Work out the finished part from the listing and answer in its coordinate system (mm). A direction names the side the tool comes from. Give positions to 0.01 mm unless a question says otherwise; leave off trailing zeros. Order: outer loops, then holes, each group sorted by start corner. A loop starts at its lowest first (then second) coordinate and runs counter-clockwise, first axis right, second up. Notation, with made-up numbers: (63, 26.25) -> (76, 26.25) arc R13 cw to (76, 47.25) -> close; hole circle Ø4 at (83, 57.5). An arc over 180 degrees is marked (long way). Use a Markdown table: item, result. Add a question column.
```python
from build123d import *

# Parameters (mm, degrees)
F1_DEPTH     = 6
F2_W         = 20.4
F2_H         = 50.2
F3_DEPTH     = 4.8
F4_R         = 8
F5_DEPTH     = 10.801
F6_R         = 2.4
F7_DEPTH     = 6.001
F8_R         = 7
F9_R         = 5
F10_T1_DEPTH = 6.0500204163


# Not quite as in the source:
# - a fillet or chamfer that OpenCascade refuses, or shapes differently, is made with other operations: its cross-section is extruded or revolved along the edge and cut away or added


with BuildPart() as f1:
    # F0 (on Top) → F1 (new body)
    with BuildSketch(Plane.XY):
        Polygon((-31, 20), (-31, 0), (31, 0), (31, 20), (17, 20), (17, 50.2), (-17, 50.2), (-17, 20), align=None)
    extrude(amount=F1_DEPTH)

    # F2 (on face) → F3 (join)
    with BuildSketch(Plane.XY.offset(6)):
        with Locations((0, 25.1)):
            Rectangle(F2_W, F2_H)
    extrude(amount=F3_DEPTH)

    # F4 (on face) → F5 (cut, through all)
    with BuildSketch(Plane.XY.offset(10.8)):
        with Locations((0, 33.2)):
            Circle(F4_R)
    extrude(amount=-F5_DEPTH, mode=Mode.SUBTRACT)

    # F6 (on face) → F7 (cut, through all)
    with BuildSketch(Plane.XY.offset(6)):
        with Locations((-25, 10)):
            Circle(F6_R)
        with Locations((25, 10)):
            Circle(F6_R)
    extrude(amount=-F7_DEPTH, mode=Mode.SUBTRACT)

    # F8
    f8_edges = [f1.edges().sort_by_distance(p)[0] for p in [
        (17, 50.2, 3),
        (-17, 50.2, 3),
    ]]
    fillet(f8_edges, radius=F8_R)

    # F9
    f9_edges = [f1.edges().sort_by_distance(p)[0] for p in [
        (-31, 20, 3),
        (31, 20, 3),
        (17, 20, 3),
        (-17, 20, 3),
    ]]
    fillet(f9_edges, radius=F9_R)

    # F10: fillet of radius 0.5 on 2 edges, made by hand

    # F10_s2 → F10_t1 (cut)
    with BuildSketch(Plane.XY.offset(6)):
        with BuildLine():
            ThreePointArc((9.7, 50.2), (10.0535533906, 50.0535533906), (10.2, 49.7))
            Line((10.2, 49.7), (10.25, 49.7))
            Line((10.25, 49.7), (10.25, 50.1971422738))
            Line((10.25, 50.1971422738), (10.2014285714, 50.2471218615))
            ThreePointArc((10.2014285714, 50.2471218615), (10, 50.25), (9.7, 50.25))
            Line((9.7, 50.25), (9.7, 50.2))
        make_face()
        with BuildLine():
            ThreePointArc((-9.7, 50.2), (-10.0535533906, 50.0535533906), (-10.2, 49.7))
            Line((-10.2, 49.7), (-10.25, 49.7))
            Line((-10.25, 49.7), (-10.25, 50.1971422738))
            Line((-10.25, 50.1971422738), (-10.2014285714, 50.2471218615))
            ThreePointArc((-10.2014285714, 50.2471218615), (-10, 50.25), (-9.7, 50.25))
            Line((-9.7, 50.25), (-9.7, 50.2))
        make_face()
    extrude(amount=F10_T1_DEPTH, mode=Mode.SUBTRACT)


solid = f1.part
```
1) Which of the six approach directions +Z, -Z, +X, -X, +Y, -Y give full straight-line access (tool end or side, diameter ignored) to faces 1 (the flat face through (18, 20, 6)), 2 (the flat face through (-18, 20, 6)), 3 (the flat face through (17, 34, 3)), 4 (the flat face through (-24, 20, 3))?
2) Determine the mould class of faces 5 (the cylindrical face through (27.29, 10.72, 3.04)), 6 (the cylindrical face through (-1.73, 25.39, 5.48)), 7 (the flat face through (0, 0, 4)), 8 (the flat face through (10.2, 25, 8)) for opening direction Y: released by +Y, released by -Y, zero draft, split by the parting line, or undercut.
3) Straight lines are drawn through the part: line 1 (Y direction, x = 25, z = 2.7); line 2 (Y direction, x = 0.5, z = 5); line 3 (Z direction, x = 21.5, y = 5). For each, find the intervals that lie inside material, in ascending order.
4) Flat-ended cylindrical pins translate along their axes: pin 1 (23.5 mm diameter, centred on x = -24.5, y = 27.5, fed in from +Z); pin 2 (1.2 mm diameter, centred on x = -25, z = 3, fed in from +Y); pin 3 (5.5 mm diameter, centred on y = 34.5, z = 9, fed in from -X). Find the tip coordinate at first contact, or state that the pin passes through.
5) The part is cut by section C-C, the plane x = 25. Determine the outline of the cut face in (y, z).
6) The part is cut by section D-D, the plane z = 4. Determine the outline of the cut face in (x, y), then the cut area to 3 significant figures.
7) The part is cut by section A-A, the plane y = 38. Determine the outline of the cut face in (x, z).
8) The part is cut by section B-B, the plane y = 10. Determine the outline of the cut face in (x, z).
A:
| question | item | result |
|---|---|---|
| 1 | face 1 | +Z, +X, +Y, -Y |
| 1 | face 2 | +Z, -X, +Y, -Y |
| 1 | face 3 | +Z, -Z, +X, +Y |
| 1 | face 4 | +Z, -Z, -X, +Y |
| 2 | face 5 | undercut |
| 2 | face 6 | undercut |
| 2 | face 7 | released by -Y |
| 2 | face 8 | zero draft |
| 3 | line 1 | 0 to 7.6, 12.4 to 20 |
| 3 | line 2 | 0 to 25.22, 41.18 to 50.2 |
| 3 | line 3 | 0 to 6 |
| 4 | pin 1 | z = 6 |
| 4 | pin 2 | y = 20 |
| 4 | pin 3 | x = -10.2 |
| 5 | outline | (0, 0) -> (7.6, 0) -> (7.6, 6) -> (0, 6) -> close; (12.4, 0) -> (20, 0) -> (20, 6) -> (12.4, 6) -> close |
| 6 | outline | (-31, 0) -> (31, 0) -> (31, 15) arc R5 ccw to (26, 20) -> (22, 20) arc R5 cw to (17, 25) -> (17, 43.2) arc R7 ccw to (10, 50.2) -> (-10, 50.2) arc R7 ccw to (-17, 43.2) -> (-17, 25) arc R5 cw to (-22, 20) -> (-26, 20) arc R5 ccw to (-31, 15) -> close; hole circle Ø4.8 at (-25, 10); hole circle Ø16 at (0, 33.2); hole circle Ø4.8 at (25, 10) |
| 6 | area | 2,010 mm^2 |
| 7 | outline | (-17, 0) -> (-6.4, 0) -> (-6.4, 10.8) -> (-10.2, 10.8) -> (-10.2, 6) -> (-17, 6) -> close; (6.4, 0) -> (17, 0) -> (17, 6) -> (10.2, 6) -> (10.2, 10.8) -> (6.4, 10.8) -> close |
| 8 | outline | (-31, 0) -> (-27.4, 0) -> (-27.4, 6) -> (-31, 6) -> close; (-22.6, 0) -> (22.6, 0) -> (22.6, 6) -> (10.2, 6) -> (10.2, 10.8) -> (-10.2, 10.8) -> (-10.2, 6) -> (-22.6, 6) -> close; (27.4, 0) -> (31, 0) -> (31, 6) -> (27.4, 6) -> close |
